from build123d import *

# Parameters (mm, degrees)
F0_W     = 57.15
F0_H     = 44.45
F1_DEPTH = 25.4
F3_DEPTH = 12.7
F5_DEPTH = 12.7


with BuildPart() as f1:
    # F0 (on Front) → F1 (new body)
    with BuildSketch(Plane.XZ):
        with Locations((28.575, 22.225)):
            Rectangle(F0_W, F0_H)
    extrude(amount=F1_DEPTH)

    # F2 (on face) → F3 (cut)
    with BuildSketch(Plane.XZ.offset(25.4)):
        Polygon((57.15, 44.45), (19.05, 44.45), (44.45, 0), (57.15, 0), align=None)
    extrude(amount=-F3_DEPTH, mode=Mode.SUBTRACT)

    # F4 (on face) → F5 (cut)
    with BuildSketch(Plane.XZ.offset(25.4)):
        with BuildLine():
            Line((36.236679, 14.373312), (23.63475, 36.426688))
            ThreePointArc((23.63475, 36.426688), (18.909026, 19.099035), (36.236679, 14.373312))
        make_face()
    extrude(amount=-F5_DEPTH, mode=Mode.SUBTRACT)


solid = f1.part
Input: part model. Units: mm. Frame: model coordinates. A direction names the side the tool comes from. Give positions to 0.01 mm unless a question says otherwise; leave off trailing zeros. Order: outer loops, then holes, each group sorted by start corner. A loop starts at its lowest first (then second) coordinate and runs counter-clockwise, first axis right, second up. Notation, with made-up numbers: M 86.5,24.25 L 137.5,24.25 A24 cw 137.5,60.25 Z; hole C 17,42 d3. An arc over 180 degrees is marked long. Answer as a JSON object with one key per item and string values.
1. First-contact query: P1, Ø20, axis at x = 47, z = 30, coming from the -Y side. Flat tip, straight axial feed; report the tip coordinate or a pass-through.
Result sheet:
{"P1": "y = -12.7"}
2. Cut plane A-A, the plane y = -22.5. Output: boundary loops of the cut face in (x, z), and give its area (3 significant figures).
Result sheet:
{"outline": "M 0,0 L 44.45,0 L 36.24,14.37 A12.7 cw 23.63,36.43 L 19.05,44.45 L 0,44.45 Z", "area": "1,160 mm²"}
3. Reachability of faces 1 (the flat face through (57.15, -6, 22)), 2 (the flat face through (21.31, -19.139, 40.495)) from +Z, -Z, +X, -X, +Y, -Y: full face, straight path, thin tool, end or side. Return the list, or none.
Result sheet:
{"face 1": "+Z, -Z, +X, +Y, -Y", "face 2": "+Z, +X, -Y"}
4. Cut plane B-B, the plane z = 25.4. Output: boundary loops of the cut face in (x, y).
Result sheet:
{"outline": "M 0,-25.4 L 17.24,-25.4 L 17.24,-12.7 L 57.15,-12.7 L 57.15,0 L 0,0 Z"}
5. Ray query, line 1 (Y direction, x = 54.5, z = 34); line 2 (Z direction, x = 20.5, y = -22.75); line 3 (X direction, y = -20.5, z = 10.5). Return the intervals inside material, ascending. Write a range as [from, to].
Result sheet:
{"line 1": "[-12.7, 0]", "line 2": "[0, 16.9], [33.9, 41.91]", "line 3": "[0, 38.45]"}
6. Pull-direction query (X, two-part tool) for faces 3 (the flat face through (40.286, -19.139, 7.287)), 4 (the flat face through (0, -13, 22)), 5 (the cylindrical face through (18.773, -19.139, 19.343)), 6 (the flat face through (28, 0, 23)); classes: +X half, -X half, draft (parallel to the pull), parting line (faces both ways), or undercut.
Result sheet:
{"face 3": "+X half", "face 4": "-X half", "face 5": "undercut", "face 6": "draft"}
7. Cut plane C-C, the plane x = 52. Output: boundary loops of the cut face in (y, z), and give its area (3 significant figures).
Result sheet:
{"outline": "M -12.7,0 L 0,0 L 0,44.45 L -12.7,44.45 Z", "area": "565 mm²"}
